The listing builds one solid part. Answer for the finished solid, in the listing's coordinates (mm). Face numbers are marked on the shaded views. A direction names the side the tool comes from. Give positions to 0.01 mm unless a question says otherwise; leave off trailing zeros. Order: outer loops, then holes, each group sorted by start corner. A loop starts at its lowest first (then second) coordinate and runs counter-clockwise, first axis right, second up. Notation, with made-up numbers: (67.5, -5.5) -> (124.5, -5.5) arc R26 ccw to (124.5, 16.5) -> close; hole circle Ø8 at (70.5, -40). An arc over 180 degrees is marked (long way). Answer as a JSON object with one key per item and string values. Group by question number.
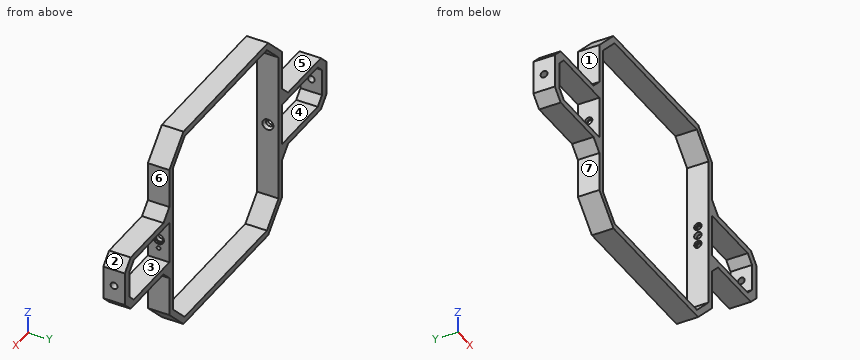
```python
from build123d import *

# Parameters (mm, degrees)
BOSS_EXTRUDE1_DEPTH      = 5.08
BOSS_EXTRUDE1_DEPTH_BACK = 5.08
SKETCH2_W                = 96.17
SKETCH2_H                = 97.44
SKETCH2_W_2              = 90.17
SKETCH2_H_2              = 91.44
SKETCH3_R                = 1.75
CUT_EXTRUDE1_DEPTH       = 108.926427255
SKETCH4_R                = 1.75
CUT_EXTRUDE2_DEPTH       = 1
SKETCH5_R                = 0.9
CUT_EXTRUDE3_DEPTH       = 107.148168613
SKETCH6_R                = 2.5
CUT_EXTRUDE4_DEPTH       = 1
BOSS_EXTRUDE2_DEPTH      = 10.16
CHAMFER1_SIZE            = 1.5
CHAMFER1_SIZE2           = 0.866025404
SKETCH9_R                = 1.625
CUT_EXTRUDE5_DEPTH       = 5
CHAMFER3_SIZE            = 10
CHAMFER4_SIZE            = 12
CHAMFER5_SIZE            = 5
CUT_EXTRUDE6_DEPTH       = 100.435864883


with BuildPart() as part:
    # Sketch2 → Boss-Extrude1 (new, two sides: drawn at the far end of the back side and taken through both)
    with BuildSketch(Plane(origin=(0, 0, 0), x_dir=(1, 0, 0), z_dir=(0, 1, 0)).offset(-BOSS_EXTRUDE1_DEPTH_BACK)):
        Rectangle(SKETCH2_W, SKETCH2_H)
        Rectangle(SKETCH2_W_2, SKETCH2_H_2, mode=Mode.SUBTRACT)
    extrude(amount=BOSS_EXTRUDE1_DEPTH + BOSS_EXTRUDE1_DEPTH_BACK)

    # Sketch3 → Cut-Extrude1 (cut, through all)
    with BuildSketch(Plane(origin=(48.085, 0, 0), x_dir=(0, 0, -1), z_dir=(1, 0, 0))):
        Circle(SKETCH3_R)
    extrude(amount=-CUT_EXTRUDE1_DEPTH, mode=Mode.SUBTRACT)

    # Sketch4 → Cut-Extrude2 (cut)
    with BuildSketch(Plane.ZY.offset(-45.085)):
        with Locations((-4.5, 0)):
            Circle(SKETCH4_R)
        with Locations(Location((4.5, 0, 0), (0, 0, 180))):
            Circle(SKETCH4_R)
    extrude(amount=-CUT_EXTRUDE2_DEPTH, mode=Mode.SUBTRACT)

    # Sketch5 → Cut-Extrude3 (cut, through all)
    with BuildSketch(Plane.ZY.offset(-46.085)):
        with Locations((-4.5, 0)):
            Circle(SKETCH5_R)
        with Locations(Location((4.5, 0, 0), (0, 0, 180))):
            Circle(SKETCH5_R)
    extrude(amount=-CUT_EXTRUDE3_DEPTH, mode=Mode.SUBTRACT)

    # Sketch6 → Cut-Extrude4 (cut)
    with BuildSketch(Plane(origin=(48.085, 0, 0), x_dir=(0, 0, -1), z_dir=(1, 0, 0))):
        Circle(SKETCH6_R)
    extrude(amount=-CUT_EXTRUDE4_DEPTH, mode=Mode.SUBTRACT)

    # Sketch8 → Boss-Extrude2 (add)
    with BuildSketch(Plane(origin=(0, 5.08, 0), x_dir=(1, 0, 0), z_dir=(0, 1, 0))):
        Polygon((48.085, -13), (86.085, -13), (86.085, 13), (48.085, 13), (48.085, 10), (78.085, 10), (78.085, -10), (48.085, -10), align=None)
        Polygon((-86.085, 13), (-86.085, -13), (-48.085, -13), (-48.085, -10), (-78.085, -10), (-78.085, 10), (-48.085, 10), (-48.085, 13), align=None)
    extrude(amount=-BOSS_EXTRUDE2_DEPTH)

    # Chamfer1
    chamfer1_edges = [part.edges().sort_by_distance(p)[0] for p in [
        (-45.085, 0, 1.75),
    ]]
    chamfer1_side = [part.faces().sort_by_distance(p)[0] for p in [
        (-46.585, 0, 1.75),
    ]]
    chamfer(chamfer1_edges, length=CHAMFER1_SIZE, length2=CHAMFER1_SIZE2, reference=chamfer1_side[0])

    # Sketch9 → Cut-Extrude5 (cut)
    with BuildSketch(Plane.ZY.offset(86.085)):
        Circle(SKETCH9_R)
    cut_extrude5 = extrude(amount=-CUT_EXTRUDE5_DEPTH, mode=Mode.SUBTRACT)

    # Mirror2: Cut-Extrude5 across plane
    add(cut_extrude5.mirror(Plane(origin=(0, 0, 0), x_dir=(0, 0, 1), z_dir=(1, 0, 0))), mode=Mode.SUBTRACT)

    # Chamfer3
    chamfer3_edges = [part.edges().sort_by_distance(p)[0] for p in [
        (45.085, 0, -45.72),
        (45.085, 0, 45.72),
        (-45.085, 0, 45.72),
        (-45.085, 0, -45.72),
    ]]
    chamfer(chamfer3_edges, length=CHAMFER3_SIZE)

    # Chamfer4
    chamfer4_edges = [part.edges().sort_by_distance(p)[0] for p in [
        (-48.085, 0, -48.72),
        (48.085, 0, -48.72),
        (48.085, 0, 48.72),
        (-48.085, 0, 48.72),
    ]]
    chamfer(chamfer4_edges, length=CHAMFER4_SIZE)

    # Chamfer5
    chamfer5_edges = [part.edges().sort_by_distance(p)[0] for p in [
        (86.085, 0, 13),
        (48.085, 0, 13),
        (48.085, 0, -13),
        (86.085, 0, -13),
        (-86.085, 0, 13),
        (-48.085, 0, 13),
        (-48.085, 0, -13),
        (-86.085, 0, -13),
    ]]
    chamfer(chamfer5_edges, length=CHAMFER5_SIZE)

    # Sketch10 → Cut-Extrude6 (cut, through all)
    with BuildSketch(Plane(origin=(0, 5.08, 0), x_dir=(1, 0, 0), z_dir=(0, 1, 0))):
        Polygon((78.085, 10), (78.085, -10), (78.428145751, -10), (82.085, -6.343145751), (82.085, 6.343145751), (78.428145751, 10), align=None)
        Polygon((-82.085, -6.343145751), (-78.428145751, -10), (-78.085, -10), (-78.085, 10), (-78.428145751, 10), (-82.085, 6.343145751), align=None)
    extrude(amount=-CUT_EXTRUDE6_DEPTH, mode=Mode.SUBTRACT)


solid = part.part
```
(1) Flat-ended cylindrical pins translate along their axes: pin 1 Ø5 at (x, y) = (70, 0) entering from -Z; pin 2 Ø4 at (y, z) = (-0.5, -0.5) entering from +X (3 decimals); pin 3 Ø1.5 at (x, y) = (50, 0) entering from +Z (3 decimals); pin 4 Ø5 at (y, z) = (-1, -26) entering from +X (3 decimals). Find the tip coordinate at first contact, or state that the pin passes through.
(2) For a pull along X with two mould halves and no side action, classify the marked faces 1, 2 and 3 as +X half, -X half, draft (parallel to the pull), parting line (faces both ways), or undercut.
(3) Find the intervals of material crossed by line 1 along Z through (x, y) = (-19, 4); line 2 along Z through (x, y) = (67, 2.5); line 3 along Y through (x, z) = (83.75, 0) (3 decimals), in increasing order. Write a range as [from, to].
(4) A cutting plane is placed at C-C (z = 0). State how many separate pieces and enclosed holes the cut face has, and give its area (3 significant figures).
(5) A cutting plane is placed at A-A (z = 24). Determine the outline of the cut face in (x, y) (3 decimals).
(6) A cutting plane is placed at B-B (x = 76). Determine the outline of the cut face in (y, z), and give its area (3 significant figures).
(7) Which of the six approach directions +Z, -Z, +X, -X, +Y, -Y give full straight-line access (tool end or side, diameter ignored) to the marked faces 4, 5, 6 and 7?
Check sheet entries:
{
 "1": {"pin 1": "stops at z = -13", "pin 2": "stops at x = 86.085", "pin 3": "stops at z = 16.835", "pin 4": "stops at x = 48.085"},
 "2": {"face 1": "-X half", "face 2": "+X half", "face 3": "undercut"},
 "3": {"line 1": "z = [-48.72, -45.72], [45.72, 48.72]", "line 2": "z = [-13, -10], [10, 13]", "line 3": "y = [-5.08, -1.625], [1.625, 5.08]"},
 "4": {"separate pieces": "8", "enclosed holes": "0", "area": "92.4 mm2"},
 "5": {"outline": "(-48.085, -5.08) -> (-45.085, -5.08) -> (-45.085, 5.08) -> (-48.085, 5.08) -> close; (45.085, -5.08) -> (48.085, -5.08) -> (48.085, 5.08) -> (45.085, 5.08) -> close"},
 "6": {"outline": "(-5.08, -13) -> (5.08, -13) -> (5.08, -10) -> (-5.08, -10) -> close; (-5.08, 10) -> (5.08, 10) -> (5.08, 13) -> (-5.08, 13) -> close", "area": "61.0 mm2"},
 "7": {"face 4": "+Y, -Y", "face 5": "+Z, -X, +Y, -Y", "face 6": "+Z, +X, +Y, -Y", "face 7": "-Z, -X, +Y, -Y"}
}
